from build123d import *

# Parameters (mm, degrees)
SKETCH1_W                  = 20.2
SKETCH1_H                  = 20.2
BOSS_EXTRUDE1_DEPTH        = 6.2
F_3_2_3_2_DIAMETER_HOLE1_D = 3.2
CUT_EXTRUDE1_START         = -2
SKETCH4_R                  = 1.6
CUT_EXTRUDE1_DEPTH         = 2


with BuildPart() as part:
    # Sketch1 → Boss-Extrude1 (new body)
    with BuildSketch(Plane(origin=(0, 6.2, 0), x_dir=(1, 0, 0), z_dir=(0, 1, 0))):
        with Locations((10.1, -12.9)):
            Rectangle(SKETCH1_W, SKETCH1_H)
    extrude(amount=-BOSS_EXTRUDE1_DEPTH)

    # Ø3.2 (3.2) Diameter Hole1 (through all)
    with Locations(Plane(origin=(0, 6.2, 0), x_dir=(1, 0, 0), z_dir=(0, 1, 0))):
        with Locations((10.1, -12.9)):
            Hole(F_3_2_3_2_DIAMETER_HOLE1_D / 2)

    # Sketch4 → Cut-Extrude1 (cut)
    with BuildSketch(Plane(origin=(0, 6.2, 0), x_dir=(1, 0, 0), z_dir=(0, 1, 0)).offset(CUT_EXTRUDE1_START)):
        Polygon((7.73670062, -10.779115898), (10.75508982, -9.792880649), (13.118389201, -11.913764751), (12.46329938, -15.020884102), (9.44491018, -16.007119351), (7.081610799, -13.886235249), align=None)
        with Locations(Location((10.1, -12.9, 0), (0, 0, 270))):
            Circle(SKETCH4_R, mode=Mode.SUBTRACT)
    extrude(amount=CUT_EXTRUDE1_DEPTH, mode=Mode.SUBTRACT)


solid = part.part
Source: CAD feature listing. Evaluate the final solid. Frame: model axes, mm. A direction names the side the tool comes from. Give positions to 0.01 mm unless a question says otherwise; leave off trailing zeros. Loops run counter-clockwise (first coordinate to the right, second up) from the corner with the lowest first, then second, coordinate; pieces in that order, holes last. Notation, with made-up numbers: (-13.5, -8) -> (12.5, -8) arc R15 cw to (12.5, 7) -> close; hole circle Ø8 at (28.5, -17.75). An arc over 180 degrees is marked (long way). Use a Markdown table: item, result. Add a question column.
1) Line query: line 1 along X through (y, z) = (2.5, 12.9); line 2 along Z through (x, y) = (10.1, 3.3); line 3 along Y through (x, z) = (11, 15). Output: solid intervals per line, ascending. Write a range as [from, to].
2) First-contact query: pin 1 (6 mm diameter, centred on x = 10, z = 14.5, fed in from +Y). Flat tip, straight axial feed; report the tip coordinate or a pass-through.
3) Pull-direction query (Z, two-part tool) for faces 1 (the face through (10, 3, 2.8)), 2 (the face through (9, 4.2, 11)), 3 (the face through (20.2, 3, 13)); classes: +Z half, -Z half, draft (parallel to the pull), parting line (faces both ways), or undercut.
4) Section query A-A, the plane y = 5. Return the cut outline in (x, z).
5) Section query C-C, the plane z = 12.9. Return the cut outline in (x, y), then the cut area to 3 significant figures.
6) Section query D-D, the plane y = 2.25. Return the cut outline in (x, z), then the cut area to 3 significant figures.
7) Section query B-B, the plane x = 11.25. Return the cut outline in (y, z).
8) Reachability of faces 4 (the face through (8, 0, 13)), 5 (the face through (11, 5.2, 15.5)) from +Z, -Z, +X, -X, +Y, -Y: full face, straight path, thin tool, end or side. Return the list, or none.
Numbers:
| question | item | result |
|---|---|---|
| 1 | line 1 | x = [0, 8.5], [11.7, 20.2] |
| 1 | line 2 | z = [2.8, 11.3], [14.5, 23] |
| 1 | line 3 | y = [0, 4.2] |
| 2 | pin 1 | stops at y = 6.2 |
| 3 | face 1 | -Z half |
| 3 | face 2 | undercut |
| 3 | face 3 | draft |
| 4 | outline | (0, 2.8) -> (20.2, 2.8) -> (20.2, 23) -> (0, 23) -> close; hole (7.08, 13.89) -> (7.74, 10.78) -> (10.76, 9.79) -> (13.12, 11.91) -> (12.46, 15.02) -> (9.44, 16.01) -> close |
| 5 | outline | (0, 0) -> (8.5, 0) -> (8.5, 4.2) -> (7.29, 4.2) -> (7.29, 6.2) -> (0, 6.2) -> close; (11.7, 0) -> (20.2, 0) -> (20.2, 6.2) -> (12.91, 6.2) -> (12.91, 4.2) -> (11.7, 4.2) -> close |
| 5 | area | 101 mm2 |
| 6 | outline | (0, 2.8) -> (20.2, 2.8) -> (20.2, 23) -> (0, 23) -> close; hole circle Ø3.2 at (10.1, 12.9) |
| 6 | area | 400 mm2 |
| 7 | outline | (0, 2.8) -> (6.2, 2.8) -> (6.2, 10.24) -> (4.2, 10.24) -> (4.2, 11.79) -> (0, 11.79) -> close; (0, 14.01) -> (4.2, 14.01) -> (4.2, 15.42) -> (6.2, 15.42) -> (6.2, 23) -> (0, 23) -> close |
| 8 | face 4 | +Z, -Z, +X, -X, -Y |
| 8 | face 5 | +Y |
